Source: CAD feature listing. Evaluate the final solid. Frame: model axes, mm. Give positions to 0.01 mm unless a question says otherwise; leave off trailing zeros. Order: outer loops, then holes, each group sorted by start corner. A loop starts at its lowest first (then second) coordinate and runs counter-clockwise, first axis right, second up. Notation, with made-up numbers: (-14, 10) - (40, 10) arc R29 cw to (40, 46) - close; hole circle Ø11 at (6, -18). An arc over 180 degrees is marked (long way). One line per item, written item: value. Start each with the question number.
from build123d import *

# Parameters (mm, degrees)
BOSS_EXTRUDE1_DEPTH = 10
SKETCH3_R           = 11.5
CUT_EXTRUDE1_DEPTH  = 11
SKETCH4_R           = 3.25
CUT_EXTRUDE2_DEPTH  = 11


with BuildPart() as part:
    # Sketch2 → Boss-Extrude1 (new body)
    with BuildSketch(Plane.XY):
        with BuildLine():
            Line((-13.5, 20), (13.5, 20))
            ThreePointArc((13.5, 20), (26.431712199, 0), (13.5, -20))
            Line((13.5, -20), (-13.5, -20))
            ThreePointArc((-13.5, -20), (-26.431712199, 0), (-13.5, 20))
        make_face()
    extrude(amount=BOSS_EXTRUDE1_DEPTH)

    # Sketch3 → Cut-Extrude1 (cut, through all)
    with BuildSketch(Plane.XY.offset(10)):
        Circle(SKETCH3_R)
    extrude(amount=-CUT_EXTRUDE1_DEPTH, mode=Mode.SUBTRACT)

    # Sketch4 → Cut-Extrude2 (cut, through all)
    with BuildSketch(Plane.XY.offset(10)):
        with Locations((-13.5, 14)):
            Circle(SKETCH4_R)
        with Locations((-13.5, -14)):
            Circle(SKETCH4_R)
        with Locations((13.5, -14)):
            Circle(SKETCH4_R)
        with Locations((13.5, 14)):
            Circle(SKETCH4_R)
    extrude(amount=-CUT_EXTRUDE2_DEPTH, mode=Mode.SUBTRACT)


solid = part.part
1. Ray query, L1, parallel to Y at x = -13.5, z = 4.25; L2, parallel to Y at x = -15.5, z = 6.5; L3, parallel to X at y = 16, z = 1.5. Return the intervals inside material, ascending.
2. Contact query for flat-ended pins moving along their axis: pin 1 Ø2 at (y, z) = (-15.5, 8) entering from -X; pin 2 Ø6 at (y, z) = (-2, 7.5) entering from -X; pin 3 Ø2 at (x, z) = (-18, 1) entering from -Y. Output: stop coordinate, or through.
3. Section A-A on x = 0. Return the cut outline in (y, z).
4. Section D-D on y = -14. Return the cut outline in (x, z), then the cut area to 3 significant figures.
5. Section C-C on z = 1. Return the cut outline in (x, y), then the cut area to 3 significant figures.
6. Draft query along Y for faces 1 (the cylindrical face through (10.253, 14.143, 5.07)), 2 (the cylindrical face through (-26.43, -0.35, 4.93)), 3 (the cylindrical face through (-1.5, 11.4, 5.1)), 4 (the flat face through (12, 0, 0)). Return one class per face: pulls with the +Y half, pulls with the -Y half, needs draft (parallel to the pull), parting line crosses it, or undercut.
7. Section B-B on y = 0. Return the cut outline in (x, z), then the cut area to 3 significant figures.
Data:
1. L1: y = -20 to -17.25, -10.75 to 10.75, 17.25 to 20
1. L2: y = -18.97 to -16.56, -11.44 to 11.44, 16.56 to 18.97
1. L3: x = -19.5 to -16.06, -10.94 to 10.94, 16.06 to 19.5
2. pin 1: stops at x = -20.95
2. pin 2: stops at x = -26.43
2. pin 3: stops at y = -18.02
3. outline: (-20, 0) - (-11.5, 0) - (-11.5, 10) - (-20, 10) - close; (11.5, 0) - (20, 0) - (20, 10) - (11.5, 10) - close
4. outline: (-21.38, 0) - (-16.75, 0) - (-16.75, 10) - (-21.38, 10) - close; (-10.25, 0) - (10.25, 0) - (10.25, 10) - (-10.25, 10) - close; (16.75, 0) - (21.38, 0) - (21.38, 10) - (16.75, 10) - close
4. area: 298 mm2
5. outline: (-13.5, -20) - (13.5, -20) arc R21.93 ccw to (13.5, 20) - (-13.5, 20) arc R21.93 ccw to start; hole circle Ø6.5 at (-13.5, -14); hole circle Ø6.5 at (-13.5, 14); hole circle Ø23 at (0, 0); hole circle Ø6.5 at (13.5, -14); hole circle Ø6.5 at (13.5, 14)
5. area: 1,280 mm2
6. face 1: undercut
6. face 2: parting line crosses it
6. face 3: undercut
6. face 4: needs draft
7. outline: (-26.43, 0) - (-11.5, 0) - (-11.5, 10) - (-26.43, 10) - close; (11.5, 0) - (26.43, 0) - (26.43, 10) - (11.5, 10) - close
7. area: 299 mm2
